The model under review builds one solid part; all positions refer to its coordinate system, in mm. A direction names the side the tool comes from. Give positions to 0.01 mm unless a question says otherwise; leave off trailing zeros. Loops run counter-clockwise (first coordinate to the right, second up) from the corner with the lowest first, then second, coordinate; pieces in that order, holes last. Notation, with made-up numbers: (61.5, 15) -> (80.5, 15) arc R19 cw to (80.5, 39) -> close; hole circle Ø10 at (89.5, 20.5). An arc over 180 degrees is marked (long way). Write each question's results on one line, items separated by ' | '. Start each with the question number.
Q1. We need section A-A (z = 1.5). Write out the cut boundary in (x, y).
Q2. Machinability: for faces 1 (the face through (-3, 48.444, -6)), 2 (the face through (-3, 48.444, 6)), 3 (the face through (-1.93, 69.21, -2.52)), 4 (the face through (1.907, 23.883, 6.057)), 5 (the face through (7, 48.444, 0)), which of the approach directions +Z, -Z, +X, -X, +Y, -Y give a long, thin tool a straight path to every point of the face, cutting with its end or side? Answer none if there is none.
Q3. We need section C-C (y = 6.35). Write out the cut boundary in (x, z) (3 decimals), plus the area to 3 significant figures.
Q4. We need section D-D (y = 58). Write out the cut boundary in (x, z), plus the area to 3 significant figures.
Q5. Wall thickness on L1, parallel to Y at x = -2.5, z = 0 (3 decimals); L2, parallel to Y at x = 3.25, z = -0.25; L3, parallel to X at y = 17.5, z = 5.5: over which ranges is each line inside the solid? List them lowest first. Write a range as [from, to].
Q6. Insertion check: pin 1 Ø1 at (x, y) = (-3.5, 42.5) entering from +Z; pin 2 Ø2 at (y, z) = (35, -2) entering from +X; pin 3 Ø1 at (x, y) = (2, 14) entering from -Z. Each pin has a flat end and moves straight along its axis. Give the tip position at first contact, or say it passes through.
Q7. We need section B-B (x = 1). Write out the cut boundary in (y, z) (3 decimals).
Q8. Mouldability with a two-part tool opening along Y and no side actions: class faces 6 (the face through (-0.09, 7.3, -3.03)), 7 (the face through (-7, 48.444, 0)), 8 (the face through (2, 62.944, -3)), 9 (the face through (5.474, 55.593, 3.219)) as released by +Y, released by -Y, zero draft, split by the parting line, or undercut.
from build123d import *

# Parameters (mm, degrees)
SKETCH1_R               = 6.35
BOSS_EXTRUDE1_DEPTH     = 48.44415
BOSS_EXTRUDE2_DEPTH     = 14.499999936
CUT_EXTRUDE1_DEPTH      = 64.687140339
CUT_EXTRUDE1_DEPTH_BACK = 64.687140339
SKETCH4_R               = 3.175
SKETCH5_R               = 3.175
BOSS_EXTRUDE3_DEPTH     = 12.7


with BuildPart() as part:
    # Sketch1 → Boss-Extrude1 (new body)
    with BuildSketch(Plane(origin=(0, 0, 0), x_dir=(1, 0, 0), z_dir=(0, 1, 0))):
        with Locations(Location((0, 0, 0), (0, 0, 270))):
            Circle(SKETCH1_R)
    extrude(amount=BOSS_EXTRUDE1_DEPTH)

    # Sketch2 → Boss-Extrude2 (add)
    with BuildSketch(Plane(origin=(0, 48.44415, 0), x_dir=(1, 0, 0), z_dir=(0, 1, 0))):
        Polygon((7.332348419, 0), (3.666174209, 6.35), (-3.666174209, 6.35), (-7.332348419, 0), (-3.666174209, -6.35), (3.666174209, -6.35), align=None)
    extrude(amount=BOSS_EXTRUDE2_DEPTH)

    # Sketch4 → Cut-Extrude1 (cut, two sides: drawn at the far end of the back side and taken through both)
    with BuildSketch(Plane(origin=(0, 0, 0), x_dir=(0, 0, -1), z_dir=(1, 0, 0)).offset(-CUT_EXTRUDE1_DEPTH_BACK)):
        with Locations((0, 6.35)):
            Circle(SKETCH4_R)
    extrude(amount=CUT_EXTRUDE1_DEPTH + CUT_EXTRUDE1_DEPTH_BACK, mode=Mode.SUBTRACT)

    # Sketch5 → Boss-Extrude3 (add)
    with BuildSketch(Plane(origin=(0, 62.944149936, 0), x_dir=(1, 0, 0), z_dir=(0, 1, 0))):
        with Locations(Location((0, 0, 0), (0, 0, 270))):
            Circle(SKETCH5_R)
    extrude(amount=BOSS_EXTRUDE3_DEPTH)


solid = part.part
Output:
1) outline: (-6.47, 48.44) -> (-6.17, 48.44) -> (-6.17, 9.15) -> (6.17, 9.15) -> (6.17, 48.44) -> (6.47, 48.44) -> (6.47, 62.94) -> (2.8, 62.94) -> (2.8, 75.64) -> (-2.8, 75.64) -> (-2.8, 62.94) -> (-6.47, 62.94) -> close; (-6.17, 0) -> (6.17, 0) -> (6.17, 3.55) -> (-6.17, 3.55) -> close
2) face 1: -Z, -X, -Y | face 2: +Z, -X, -Y | face 3: +Y | face 4: -Y | face 5: +X, -Y
3) outline: (-5.499, -3.175) arc R6.35 ccw to (5.499, -3.175) -> close; (-5.499, 3.175) -> (5.499, 3.175) arc R6.35 ccw to start | area: 49.5 mm2
4) outline: (-7.33, 0) -> (-3.67, -6.35) -> (3.67, -6.35) -> (7.33, 0) -> (3.67, 6.35) -> (-3.67, 6.35) -> close | area: 140 mm2
5) L1: [0, 3.175], [9.525, 75.644] | L2: [0, 3.18], [9.52, 62.94] | L3: [-3.17, 3.17]
6) pin 1: z = 5.6 | pin 2: x = 6.27 | pin 3: z = -6.17
7) outline: (0, -6.271) -> (48.444, -6.271) -> (48.444, -6.35) -> (62.944, -6.35) -> (62.944, -3.013) -> (75.644, -3.013) -> (75.644, 3.013) -> (62.944, 3.013) -> (62.944, 6.35) -> (48.444, 6.35) -> (48.444, 6.271) -> (0, 6.271) -> close; hole circle Ø6.35 at (6.35, 0)
8) face 6: undercut | face 7: released by -Y | face 8: released by +Y | face 9: zero draft
